```python
from build123d import *

# Parameters (mm, degrees)
SKETCH2_R           = 31.85
BOSS_EXTRUDE1_DEPTH = 6.5
SKETCH3_W           = 6
SKETCH3_H           = 6
CUT_EXTRUDE1_DEPTH  = 6.5
CHAMFER1_SIZE       = 6
CHAMFER1_SIZE2      = 3.057152697
SKETCH5_R           = 1.5
CUT_EXTRUDE2_DEPTH  = 56.252556502
SKETCH6_R           = 2.5
CUT_EXTRUDE3_DEPTH  = 3
CHAMFER3_SIZE       = 1.5
BOSS_EXTRUDE2_DEPTH = 1


with BuildPart() as part:
    # Sketch2 → Boss-Extrude1 (new body)
    with BuildSketch(Plane.XY.offset(-25.5)):
        Circle(SKETCH2_R)
    extrude(amount=-BOSS_EXTRUDE1_DEPTH)

    # Sketch3 → Cut-Extrude1 (cut)
    with BuildSketch(Plane(origin=(0, 0, -32), x_dir=(-1, 0, 0), z_dir=(0, 0, -1))):
        with Locations((-21, 0)):
            Rectangle(SKETCH3_W, SKETCH3_H)
        Rectangle(SKETCH3_W, SKETCH3_H)
    extrude(amount=-CUT_EXTRUDE1_DEPTH, mode=Mode.SUBTRACT)

    # Chamfer1
    chamfer1_edges = [part.edges().sort_by_distance(p)[0] for p in [
        (3, 0, -32),
        (0, -3, -32),
        (-3, 0, -32),
        (0, 3, -32),
        (24, 0, -32),
        (21, -3, -32),
        (18, 0, -32),
        (21, 3, -32),
    ]]
    chamfer1_side = [part.faces().sort_by_distance(p)[0] for p in [
        (-30.949145961, 0, -32),
    ]]
    chamfer(chamfer1_edges, length=CHAMFER1_SIZE, length2=CHAMFER1_SIZE2, reference=chamfer1_side[0])

    # Sketch5 → Cut-Extrude2 (cut, through all)
    with BuildSketch(Plane.XY):
        with Locations((-17.971861544, -17.500238124)):
            Circle(SKETCH5_R)
        with Locations((17.971861544, -17.500238124)):
            Circle(SKETCH5_R)
        with Locations((17.971861544, 17.500238124)):
            Circle(SKETCH5_R)
        with Locations((-17.971861544, 17.500238124)):
            Circle(SKETCH5_R)
    extrude(amount=-CUT_EXTRUDE2_DEPTH, mode=Mode.SUBTRACT)

    # Sketch6 → Cut-Extrude3 (cut)
    with BuildSketch(Plane.XY.offset(-32)):
        with Locations((-17.971861544, -17.500238124)):
            Circle(SKETCH6_R)
        with Locations(Location((17.971861544, -17.500238124, 0), (0, 0, 180))):
            Circle(SKETCH6_R)
        with Locations((17.971861544, 17.500238124)):
            Circle(SKETCH6_R)
        with Locations(Location((-17.971861544, 17.500238124, 0), (0, 0, 180))):
            Circle(SKETCH6_R)
    extrude(amount=CUT_EXTRUDE3_DEPTH, mode=Mode.SUBTRACT)

    # Chamfer3
    chamfer3_edges = [part.edges().sort_by_distance(p)[0] for p in [
        (-31.85, 0, -25.5),
    ]]
    chamfer(chamfer3_edges, length=CHAMFER3_SIZE)

    # Sketch7 → Boss-Extrude2 (add)
    with BuildSketch(Plane.XY.offset(-25.5)):
        Polygon((-1.25, -2), (-2, -2), (-2, 2), (-1.25, 2), (-1.25, 3), (-3, 3), (-3, -3), (-1.25, -3), align=None)
        Polygon((1.2909118, -3), (3, -3), (3, 3), (1.2909118, 3), (1.2909118, 2), (2, 2), (2, -2), (1.2909118, -2), align=None)
        Polygon((19.75, -2), (19, -2), (19, 2), (19.75, 2), (19.75, 3), (18, 3), (18, -3), (19.75, -3), align=None)
        Polygon((22.2909118, -3), (24, -3), (24, 3), (22.2909118, 3), (22.2909118, 2), (23, 2), (23, -2), (22.2909118, -2), align=None)
    extrude(amount=-BOSS_EXTRUDE2_DEPTH)


solid = part.part
```
Geometry: final body of the model. Coordinates: model frame, mm. A direction names the side the tool comes from. Coordinates: 2 decimals unless noted, no trailing zeros. Order: outer loops, then holes, each group sorted by start corner. A loop starts at its lowest first (then second) coordinate and runs counter-clockwise, first axis right, second up. Notation, with made-up numbers: (-33.5, 39) - (19.5, 39) arc R22 ccw to (19.5, 58) - close; hole circle Ø11 at (23.25, 52.5). An arc over 180 degrees is marked (long way). Return JSON: item names as keys, results as strings. Group by question number.
1. Pin query (flat end, axial travel): pin 1 (12 mm diameter, centred on x = -1.5, y = -1.5, fed in from -Z); pin 2 (0.5 mm diameter, centred on y = 2.5, z = -26, fed in from +X); pin 3 (4 mm diameter, centred on x = -17.97, y = -17.5, fed in from -Z). Return the tip coordinate at first contact, or that it passes through.
2. Set-up query: faces 4 (the face through (3, 0, -28)), 5 (the face through (0, -6, -25.5)). Return all of +Z, -Z, +X, -X, +Y, -Y with unobstructed straight access to the full face (end or side cutting, diameter ignored); none if empty.
3. Cut plane A-A (y = 0). Output: boundary loops of the cut face in (x, z).
4. Material intervals for line 1 along X through (y, z) = (1.5, -30); line 2 along X through (y, z) = (-1, -25.75); line 3 along Z through (x, y) = (-16.5, -19), sorted ascending. Write a range as [from, to].
5. Pull-direction query (X, two-part tool) for faces 1 (the face through (-15, 0, -32)), 2 (the face through (21, 3, -28)), 3 (the face through (30.38, 9.57, -29.46)); classes: pulls with the +X half, pulls with the -X half, needs draft (parallel to the pull), parting line crosses it, or undercut.
6. Cut plane C-C (z = -28). Output: boundary loops of the cut face in (x, y), plus the area to 3 significant figures.
7. Cut plane B-B (x = 0). Output: boundary loops of the cut face in (y, z), plus the area to 3 significant figures.
Resolved:
{
 "1": {"pin 1": "stops at z = -31.24", "pin 2": "stops at x = 31", "pin 3": "stops at z = -29"},
 "2": {"face 4": "-Z", "face 5": "+Z, +X, -X, +Y, -Y"},
 "3": {"outline": "(-31.85, -32) - (-9, -32) - (-3, -28.94) - (-3, -26.5) - (-2, -26.5) - (-2, -25.5) - (-30.35, -25.5) - (-31.85, -27) - close; (2, -26.5) - (3, -26.5) - (3, -28.94) - (9, -32) - (12, -32) - (18, -28.94) - (18, -26.5) - (19, -26.5) - (19, -25.5) - (2, -25.5) - close; (23, -26.5) - (24, -26.5) - (24, -28.94) - (30, -32) - (31.85, -32) - (31.85, -27) - (30.35, -25.5) - (23, -25.5) - close"},
 "4": {"line 1": "x = [-31.81, -5.07], [5.07, 15.93], [26.07, 31.81]", "line 2": "x = [-30.58, -2], [2, 19], [23, 30.58]", "line 3": "z = [-29, -25.5]"},
 "5": {"face 1": "needs draft", "face 2": "undercut", "face 3": "parting line crosses it"},
 "6": {"outline": "circle Ø63.7 at (0, 0); hole circle Ø3 at (-17.97, -17.5); hole circle Ø3 at (-17.97, 17.5); hole (-3, -3) - (3, -3) - (3, 3) - (-3, 3) - close; hole circle Ø3 at (17.97, -17.5); hole circle Ø3 at (17.97, 17.5); hole (18, -3) - (24, -3) - (24, 3) - (18, 3) - close", "area": "3,090 mm²"},
 "7": {"outline": "(-31.85, -32) - (-9, -32) - (-3, -28.94) - (-3, -25.5) - (-30.35, -25.5) - (-31.85, -27) - close; (3, -28.94) - (9, -32) - (31.85, -32) - (31.85, -27) - (30.35, -25.5) - (3, -25.5) - close", "area": "354 mm²"}
}
